Autodesk Inventor part; units mm, degrees
ref_plane "Work Plane2" through (-78.4932, -111.5319, 135) normal (0, 0, -1) x (0, 1, 0)
ref_plane "YZ Plane" through (0, 0, 0) normal (1, 0, 0) x (0, 1, 0)
ref_plane "XZ Plane" through (0, 0, 0) normal (0, 1, 0) x (-1, 0, 0)
ref_plane "Work Plane1" through (0, 0, 0) normal (0, 0, 1) x (1, 0, 0)
sketch "Sketch1" plane through (0, 0, 0) normal (0, 0, 1) x (1, 0, 0)
  circle A0 centre (-55.8916, -14.7421) radius 1.397
  circle A1 centre (-83.8916, 18.2579) radius 1.397 construction
  circle A2 centre (-83.8916, -14.7421) radius 1.397 construction
  circle A3 centre (-55.8916, 18.2579) radius 1.397
  circle A4 centre (2.1895, 105.4705) radius 2.159
  circle A5 centre (-2.169, -104.4843) radius 2.159
  circle A6 centre (60.6164, 51.7463) radius 2.159
  circle A7 centre (-58.4167, 54.2173) radius 2.159
  arc A8 (6.6818, 105.2084) -> (-2.3099, 105.3951) centre (2.1895, 105.4705) ccw
  arc A9 (-2.3099, 105.3951) -> (-57.5952, 58.6417) centre (0.9442, 45.4834) ccw
  arc A10 (-57.5952, 58.6417) -> (-59.0718, 49.7652) centre (-58.4167, 54.2173) ccw
  line L0 (-59.0718, 49.7652) -> (-63.1925, 21.7579)
  line L1 (-87.8916, 21.7579) -> (-63.1925, 21.7579)
  line L2 (-87.8916, -18.2421) -> (-87.8916, 21.7579)
  line L3 (-87.8916, -18.2421) -> (-74.0344, -26.2425)
  arc A11 (-74.0344, -26.2425) -> (-70.4822, -28.7807) centre (-69.9706, -24.3098) ccw
  arc A12 (-70.4822, -28.7807) -> (-6.6627, -104.2463) centre (-0.7162, -34.4994) ccw
  arc A13 (-6.6627, -104.2463) -> (2.3307, -104.433) centre (-2.169, -104.4843) ccw
  arc A14 (2.3307, -104.433) -> (69.2271, -31.6809) centre (-0.7162, -34.4994) ccw
  arc A15 (69.2271, -31.6809) -> (68.4317, -22.7173) centre (68.9014, -27.1927) ccw
  line L4 (68.4317, -22.7173) -> (61.0862, 47.2708)
  arc A16 (61.0862, 47.2708) -> (59.9792, 56.2009) centre (60.6164, 51.7463) ccw
  arc A17 (59.9792, 56.2009) -> (6.6818, 105.2084) centre (0.9442, 45.4834) ccw
  circle A18 centre (-69.9706, -24.3098) radius 2.159
  circle A19 centre (68.9014, -27.1927) radius 2.159
  circle A20 centre (0.9442, 45.4834) radius 17.5
  circle A21 centre (-0.7162, -34.4994) radius 17.5
  circle A22 centre (-66.7556, 10.6536) radius 4
  circle A23 centre (-75.8916, -7.1378) radius 4
  circle A24 centre (68.9014, -27.1927) radius 2.159 construction
  circle A25 centre (60.6164, 51.7463) radius 2.159 construction
  circle A26 centre (-2.169, -104.4843) radius 2.159 construction
  circle A27 centre (2.1895, 105.4705) radius 2.159 construction
  arc A28 (6.6818, 105.2084) -> (-2.3099, 105.3951) centre (2.1895, 105.4705) ccw construction
  arc A29 (59.9792, 56.2009) -> (6.6818, 105.2084) centre (0.9442, 45.4834) ccw construction
  arc A30 (61.0862, 47.2708) -> (59.9792, 56.2009) centre (60.6164, 51.7463) ccw construction
  line L5 (61.0862, 47.2708) -> (68.4317, -22.7173) construction
  arc A31 (69.2271, -31.6809) -> (68.4317, -22.7173) centre (68.9014, -27.1927) ccw construction
  arc A32 (2.3307, -104.433) -> (69.2271, -31.6809) centre (-0.7162, -34.4994) ccw construction
  arc A33 (-6.6627, -104.2463) -> (2.3307, -104.433) centre (-2.169, -104.4843) ccw construction
  line L6 (-6.6627, -104.2463) -> (-6.5797, -100.2463) construction
  arc A34 (-6.5797, -100.2463) -> (64.9314, -27.6121) centre (-0.7162, -34.4994) ccw construction
  line L7 (64.9314, -27.6121) -> (56.6497, 51.3276) construction
  arc A35 (56.6497, 51.3276) -> (-2.393, 101.3951) centre (0.9442, 45.4834) ccw construction
  line L8 (-2.393, 101.3951) -> (-2.3099, 105.3951) construction
  line L9 (-6.6627, -104.2463) -> (-6.5797, -100.2463)
  line L10 (-2.393, 101.3951) -> (-2.3099, 105.3951)
  arc A36 (-2.393, 101.3951) -> (-54.4704, 53.6367) centre (0.9442, 45.4834) ccw
  line L11 (-54.4704, 53.6367) -> (-59.6022, 18.7579)
  line L12 (-59.6022, 18.7579) -> (-84.8916, 18.7579)
  line L13 (-84.8916, 18.7579) -> (-84.8916, -12.0475)
  arc A37 (-66.7218, -35.0506) -> (-6.5797, -100.2463) centre (-0.7162, -34.4994) ccw
  arc A38 (-66.8117, -24.2835) -> (-68.3911, -21.5741) centre (-69.9706, -24.3098) ccw
  line L14 (-66.7218, -35.0506) -> (-66.8117, -24.2835)
  line L15 (-84.8916, -12.0475) -> (-68.3911, -21.5741)
  point P0 (0, 0)
  dimension "d0" = 1
  dimension "d1" = 3
  dimension "d2" = 3
extrude "Extrusion1" add sketch "Sketch1" along normal blind 125 contours L10 A36 L11 L12 L13 L15 A38 L14 A37 L9 A12 A11 L3 L2 L1 L0 A10 A9
sketch "Sketch2" plane through (0, 0, 125) normal (0, 0, 1) x (1, 0, 0)
  circle A0 centre (-69.9706, -24.3098) radius 2.159
  circle A1 centre (-58.4167, 54.2173) radius 2.159
  arc A2 (-2.3099, 105.3951) -> (-57.5952, 58.6417) centre (0.9442, 45.4834) ccw
  arc A3 (-57.5952, 58.6417) -> (-59.0718, 49.7652) centre (-58.4167, 54.2173) ccw
  line L0 (-59.0718, 49.7652) -> (-63.1925, 21.7579)
  line L1 (-63.1925, 21.7579) -> (-87.8916, 21.7579)
  line L2 (-87.8916, 21.7579) -> (-87.8916, -18.2421)
  line L3 (-87.8916, -18.2421) -> (-74.0344, -26.2425)
  arc A4 (-74.0344, -26.2425) -> (-70.4822, -28.7807) centre (-69.9706, -24.3098) ccw
  arc A5 (-70.4822, -28.7807) -> (-6.6627, -104.2463) centre (-0.7162, -34.4994) ccw
  line L4 (-6.6627, -104.2463) -> (-6.5797, -100.2463)
  arc A6 (-66.7218, -35.0506) -> (-6.5797, -100.2463) centre (-0.7162, -34.4994) ccw
  line L5 (-66.7218, -35.0506) -> (-66.8117, -24.2835)
  arc A7 (-66.8117, -24.2835) -> (-68.3911, -21.5741) centre (-69.9706, -24.3098) ccw
  line L6 (-68.3911, -21.5741) -> (-84.8916, -12.0475)
  line L7 (-84.8916, -12.0475) -> (-84.8916, 18.7579)
  line L8 (-84.8916, 18.7579) -> (-59.6022, 18.7579)
  line L9 (-59.6022, 18.7579) -> (-54.4704, 53.6367)
  arc A8 (-2.393, 101.3951) -> (-54.4704, 53.6367) centre (0.9442, 45.4834) ccw
  line L10 (-2.393, 101.3951) -> (-2.3099, 105.3951)
  circle A9 centre (-66.7556, 10.6536) radius 4
  circle A10 centre (-75.8916, -7.1378) radius 4
  line L11 (-66.7218, -35.0506) -> (-66.8117, -24.2835)
  line L12 (-59.6022, 18.7579) -> (-66.8117, -24.2835)
  point P0 (0, 0)
ref_plane "Work Plane2" through (-78.4932, -111.5319, 135) normal (0, 0, -1) x (0, 1, 0)
extrude "Extrusion2" add sketch "Sketch2" along normal up to surface (10 mm away)
properties part number "case top half"
Model file for the job. Use its own axes, mm. A direction names the side the tool comes from. Give positions to 0.01 mm unless a question says otherwise; leave off trailing zeros. Write each loop counter-clockwise with the first axis right and the second up, starting at its lowest first coordinate (ties: lowest second). Pieces come first, ordered by that corner, then holes. Notation, with made-up numbers: M 82,58 L 136,58 A33 ccw 136,86 Z; hole C 27.5,40.5 d5. An arc over 180 degrees is marked long. Use a Markdown table: item, result.
1) Cut at C-C (x = -39.5). List the corners of the cut face in (y, z), and give its area (3 significant figures).
Responses:
| item | result |
|---|---|
| outline | M -92.77,0 L -87.91,0 L -87.91,135 L -92.77,135 Z; M 84.23,0 L 89.8,0 L 89.8,135 L 84.23,135 Z |
| area | 1,410 mm2 |
2) Drill centre lines: line 1 (Y direction, x = -71.5, z = 69); line 2 (Z direction, x = -66, y = 1); line 3 (X direction, y = -6.5, z = 54.5). Where is each one in solid material? Low to high. Write a range as from..to.
Responses:
| item | result |
|---|---|
| line 1 | y = -28.54..-25.83, -22.79..-19.78, 18.76..21.76 |
| line 2 | z = 125..135 |
| line 3 | x = -87.89..-84.89 |
3) Cut at A-A (x = -9). List the corners of the cut face in (y, z), and give its area (3 significant figures).
Responses:
| item | result |
|---|---|
| outline | M -104.01,0 L -99.99,0 L -99.99,135 L -104.01,135 Z; M 100.6,0 L 104.65,0 L 104.65,135 L 100.6,135 Z |
| area | 1,090 mm2 |
4) Pin check, flat tips, straight feed: pin 1 (6 mm diameter, centred on y = -18, z = 78.5, fed in from +X); pin 2 (1 mm diameter, centred on x = -16.5, z = 119, fed in from -Y); pin 3 (1.5 mm diameter, centred on y = 69.5, z = 62, fed in from +X); pin 4 (4 mm diameter, centred on x = -58.42, y = 54.22, fed in from -Z). Stop position of each tip, or through.
Responses:
| item | result |
|---|---|
| pin 1 | stops at x = -69.39 |
| pin 2 | stops at y = -102.81 |
| pin 3 | stops at x = -49.29 |
| pin 4 | passes through |
5) Cut at B-B (z = 47.5). List the corners of the cut face in (x, y).
Responses:
| item | result |
|---|---|
| outline | M -87.89,-18.24 L -74.03,-26.24 A4.5 ccw -70.48,-28.78 A70 ccw -6.66,-104.25 L -6.58,-100.25 A66.01 cw -66.72,-35.05 L -66.81,-24.28 A3.16 ccw -68.39,-21.57 L -84.89,-12.05 L -84.89,18.76 L -59.6,18.76 L -54.47,53.64 A56.01 cw -2.39,101.4 L -2.31,105.4 A60 ccw -57.6,58.64 A4.5 ccw long -59.07,49.77 L -63.19,21.76 L -87.89,21.76 Z; hole C -69.97,-24.31 d4.32; hole C -58.42,54.22 d4.32 |
6) Cut at D-D (y = 40.5). List the corners of the cut face in (x, z).
Responses:
| item | result |
|---|---|
| outline | M -60.43,0 L -56.4,0 L -56.4,135 L -60.43,135 Z |
7) Pull direction Y, two halves, no side cores. Call faces 1 (the flat face through (-63.156, -2.462, 129.93)), 2 (the flat face through (-64, 1, 135)), 3 (the flat face through (-76, 21.758, 67)): +Y half, -Y half, draft (parallel to the pull), parting line (faces both ways), or undercut.
Responses:
| item | result |
|---|---|
| face 1 | undercut |
| face 2 | draft |
| face 3 | +Y half |
8) Tool access for faces 4 (the flat face through (-76.76, -16.74, 61.62)), 5 (the flat face through (-61.103, 35.958, 66.555)), 6 (the cylindrical face through (-37.306, 86.4, 66.555)): list every direction of +Z, -Z, +X, -X, +Y, -Y with a clear straight run to the whole face (end or side of a thin tool).
Responses:
| item | result |
|---|---|
| face 4 | -Z, +X |
| face 5 | +Z, -Z, -X |
| face 6 | +Z, -Z, +X |
